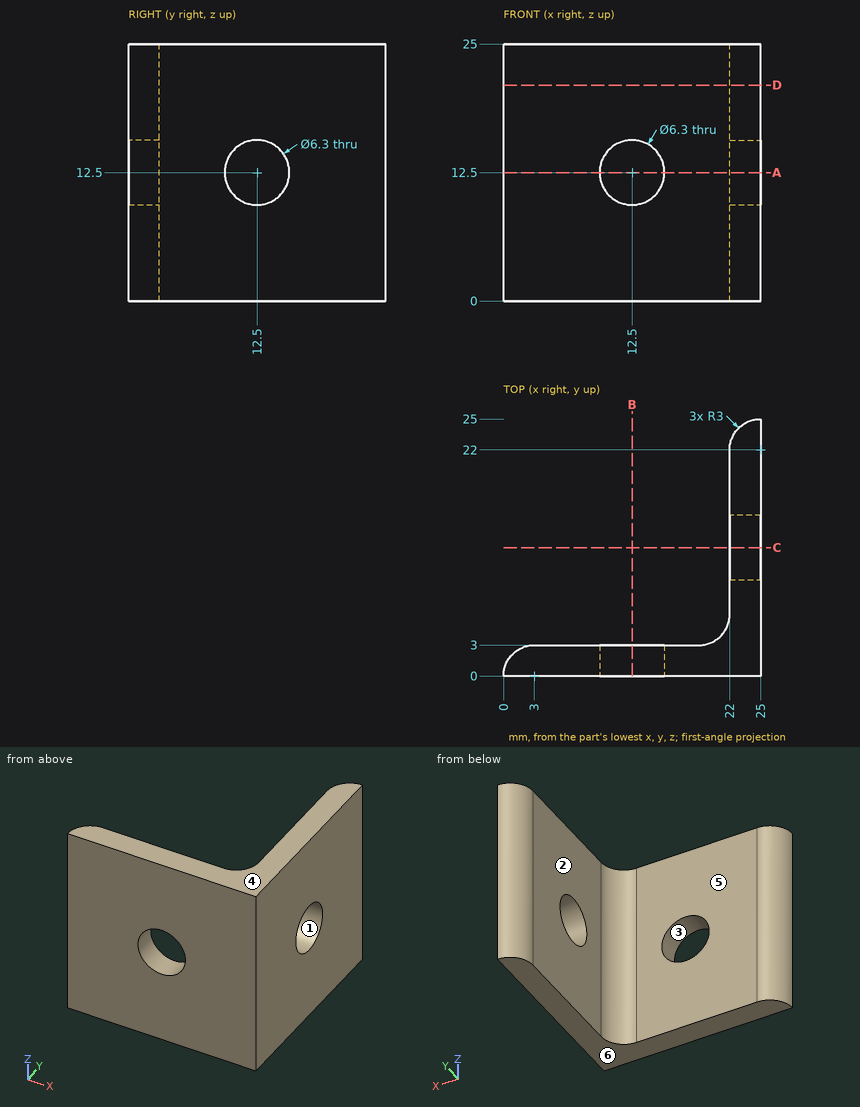
Could you check a few things on this drawing? It's one solid part, dimensions in mm from its lowest x, y, z. A direction names the side the tool comes from. Round coordinates to 2 decimals unless told otherwise and drop trailing zeros. Write each loop counter-clockwise with the first axis right and the second up, starting at its lowest first coordinate (ties: lowest second). Pieces come first, ordered by that corner, then holes.
Q1. If we mould it in two halves opening along Z, with no side actions, what happens to the marked faces 1, 2, 3 and 4? For each: +Z half, -Z half, draft (parallel to the pull), parting line (faces both ways), or undercut.
Q2. Which directions (+Z, -Z, +X, -X, +Y, -Y) give clear straight access to the entire face, cutting with the end or side of a thin tool? Please do the marked faces 5 and 6.
Q3. If we section it at A-A on z = 12.5: Write out the boundary of the cut face in (x, y), plus the area to 3 significant figures.
Q4. Please list where these lines run through material, in increasing order: probe 1 along Z at (x, y) = (24, 12.5); probe 2 along Y at (x, z) = (15.75, 2.5); probe 3 along X at (y, z) = (22, 1.5).
Q5. Will these pins go through, and if not, where does the flat tip stop? P1, Ø7, axis at x = 12.5, z = 12.5, coming from the +Y side; P2, Ø5.5, axis at y = 12.5, z = 12.5, coming from the -X side; P3, Ø1.5, axis at y = 7, z = 9, coming from the -X side; P4, Ø6, axis at x = 4, z = 8.5, coming from the -Y side.
Q6. If we section it at B-B on x = 12.5: Write out the boundary of the cut face in (y, z), plus the area to 3 significant figures.
Q7. If we section it at D-D on z = 21: Write out the boundary of the cut face in (x, y), plus the area to 3 significant figures.
Q8. If we section it at C-C on y = 12.5: Write out the boundary of the cut face in (x, z).
Answer below:
1. face 1: undercut
1. face 2: draft
1. face 3: undercut
1. face 4: +Z half
2. face 5: +Z, -Z, -X, +Y
2. face 6: -Z, +X, -X, +Y, -Y
3. outline: (0, 0) - (9.35, 0) - (9.35, 3) - (3, 3) arc R3 ccw to start; (15.65, 0) - (25, 0) - (25, 9.35) - (22, 9.35) - (22, 6) arc R3 cw to (19, 3) - (15.65, 3) - close; (22, 15.65) - (25, 15.65) - (25, 25) arc R3 ccw to (22, 22) - close
3. area: 101 mm2
4. probe 1: z = 0 to 9.35, 15.65 to 25
4. probe 2: y = 0 to 3
4. probe 3: x = 22 to 25
5. P1: stops at y = 3
5. P2: passes through
5. P3: stops at x = 22
5. P4: stops at y = 0
6. outline: (0, 0) - (3, 0) - (3, 9.35) - (0, 9.35) - close; (0, 15.65) - (3, 15.65) - (3, 25) - (0, 25) - close
6. area: 56.1 mm2
7. outline: (0, 0) - (25, 0) - (25, 25) arc R3 ccw to (22, 22) - (22, 6) arc R3 cw to (19, 3) - (3, 3) arc R3 ccw to start
7. area: 139 mm2
8. outline: (22, 0) - (25, 0) - (25, 9.35) - (22, 9.35) - close; (22, 15.65) - (25, 15.65) - (25, 25) - (22, 25) - close
